Part model, mm, in its own coordinate system. A direction names the side the tool comes from. Round coordinates to 2 decimals unless told otherwise and drop trailing zeros. Loops run counter-clockwise (first coordinate to the right, second up) from the corner with the lowest first, then second, coordinate; pieces in that order, holes last.
1) 3-axis set-ups, long thin cutter, end or side, ignore diameter. For faces 4 (the flat face through (302.45, -195.1, -14.95)), 5 (the flat face through (304.884, -195.453, -28.203)): which of +Z, -Z, +X, -X, +Y, -Y reach the whole face in a straight line?
2) Band-saw the part on C-C, the plane y = -201.5. Write the cut outline in (x, z), then the cut area to 3 significant figures.
3) Band-saw the part on A-A, the plane z = -4. Write the cut outline in (x, y).
4) Probe line 1 (X direction, y = -198.75, z = -15.5); line 2 (X direction, y = -191.75, z = -21.5); line 3 (Z direction, x = 314, y = -187.75). List the from-to ranges inside material, lowest first.
5) Band-saw the part on B-B, the plane z = -17.5. Write the cut outline in (x, y).
6) Drop flat-ended pins along their axis: P1, Ø10, axis at y = -191, z = -7, coming from the +X side; P2, Ø8, axis at x = 329, y = -199.5, coming from the -Z side; P3, Ø6, axis at x = 318, y = -192, coming from the +Z side. Give the stop position or say it passes through.
7) Band-saw the part on D-D, the plane x = 308. Write the cut outline in (y, z), then the cut area to 3 significant figures.
8) Mould opens along X. For faces 1 (the flat face through (321.5, -182.575, -20.2)), 2 (the flat face through (302.59, -195.1, -25.1)), 3 (the flat face through (302.786, -195.453, -10.139)) say: +X half, -X half, draft (parallel to the pull), parting line (faces both ways), or undercut.
Autodesk Inventor part; units mm, degrees
ref_plane "YZ Plane" through (0, 0, 0) normal (1, 0, 0) x (0, 1, 0)
ref_plane "XZ Plane" through (0, 0, 0) normal (0, 1, 0) x (-1, 0, 0)
ref_plane "XY Plane" through (0, 0, 0) normal (0, 0, 1) x (1, 0, 0)
ref_plane "Work Plane1" through (330.6234, -207.9752, -19.9742) normal (0, 1, 0) x (-1, 0, -0.0009)
sketch "Sketch1" plane through (330.6234, -207.9752, -19.9742) normal (0, 1, 0) x (-1, 0, -0.0009)
  circle A0 centre (33.1445, -22.86) radius 4
  circle A1 centre (33.1445, -22.86) radius 4
  circle A2 centre (33.1445, -22.86) radius 4
  line L0 (20.4234, -0.007) -> (20.405, 19.993)
  line L1 (660.8047, 20.5832) -> (0.405, 19.9746)
  line L2 (0.4234, -0.0254) -> (0.405, 19.9746)
  line L3 (0.4234, -0.0254) -> (660.8231, 0.5832)
  line L4 (660.8047, 20.5832) -> (660.8231, 0.5832)
  line L5 (0.405, 19.9746) -> (-7.215, 19.9746)
  line L6 (0.405, 19.9746) -> (0.4234, -0.0254)
  line L7 (0.4234, -0.0254) -> (20.4234, -0.007)
  line L8 (20.4234, -0.007) -> (20.405, 19.993)
  line L9 (35.0462, 0.0065) -> (20.405, 19.993)
  line L10 (-7.215, 19.9746) -> (-7.215, 0.0065)
  line L11 (-7.215, 0.0065) -> (-7.215, -5.0735)
  line L12 (-7.215, -5.0735) -> (20.405, -5.0735)
  line L13 (20.405, -5.0735) -> (31.2395, -11.4268)
  arc A3 (35.0462, -19.341) -> (31.2395, -19.3428) centre (33.1445, -22.86) ccw
  line L14 (31.2395, -19.3428) -> (31.2395, -11.4268)
  line L15 (35.0462, -19.341) -> (35.0462, 0.0065)
  line L16 (20.405, 19.993) -> (20.4234, -0.007)
  line L17 (0.4234, -0.0254) -> (20.4234, -0.007)
  point P0 (330.6048, 20.2789)
  dimension "d0" = 7.62
  dimension "d3" = 5.08
extrude "Extrusion1" add sketch "Sketch1" along normal blind 25.4 contours A0 L14 L13 L12 L11 L10 L5 L2 L3 L15 | L3 L0 L9
sketch "Sketch2" plane through (337.8431, -207.9752, -25.0411) normal (1, 0, 0.0009) x (0.0009, 0, -1)
  line L0 (14.2693, 0) -> (14.2693, 25.4)
  line L1 (-5.0481, 0) -> (-5.0481, 25.4)
  line L2 (-25.0481, 25.4) -> (0, 25.4)
  line L3 (-25.0481, 0) -> (-25.0481, 25.4)
  line L4 (-5.0481, 25.4) -> (-25.0481, 25.4)
  line L5 (-15.0481, 25.4) -> (-15.0481, 12.7)
  circle A0 centre (-15.0481, 12.7) radius 2.5
  point P0 (-25.3524, 207.9752)
  dimension "d6" = 5
extrude "Extrusion2" cut sketch "Sketch2" against normal blind 25.4
sketch "Sketch3" plane through (330.6234, -182.5752, -19.9742) normal (0, 1, 0) x (1, 0, 0.0009)
  line L0 (-20.4234, 0.007) -> (-0.4234, 0.0254)
  line L1 (-0.4234, 0.0254) -> (-0.405, -19.9746)
  line L2 (-0.405, -19.9746) -> (7.215, -19.9746)
  line L3 (7.215, -19.9746) -> (7.215, 5.0735)
  line L4 (7.215, 5.0735) -> (-20.405, 5.0735)
  line L5 (-20.405, 5.0735) -> (-31.2395, 11.4268)
  line L6 (-31.2395, 11.4268) -> (-31.2395, 19.3428)
  arc A0 (-35.0462, 19.341) -> (-31.2395, 19.3428) centre (-33.1445, 22.86) ccw
  line L7 (-35.0462, 19.341) -> (-35.0462, -0.0065)
  line L8 (-35.0462, -0.0065) -> (-20.405, -19.993)
  line L9 (-20.405, -19.993) -> (-20.4234, 0.007)
  line L10 (-32.7964, 8.2501) -> (-32.7964, 0.8179)
  line L11 (-32.7964, 0.8179) -> (-23.4059, -11.0873)
  line L12 (-23.4059, -11.0873) -> (-23.4059, 2.0332)
  line L13 (-23.4059, 2.0332) -> (-32.7964, 8.2501)
  point P0 (-330.6048, -20.2789)
extrude "Extrusion3" cut sketch "Sketch3" against normal blind 50.8 contours L13 L12 L11 L10
sketch "Sketch4" plane through (337.82, -207.9752, 0.007) normal (-0.0009, 0, 1) x (1, 0, 0.0009)
  point P0 (-337.8199, 207.9752)
sketch "Sketch5" plane through (330.6234, -182.5752, -19.9742) normal (0, 1, 0) x (1, 0, 0.0009)
  line L0 (-0.405, -19.9746) -> (7.215, -19.9746)
  line L1 (-0.4234, 0.0254) -> (-0.405, -19.9746)
  line L2 (-0.405, -19.9746) -> (-1.675, -19.9746)
  line L3 (-0.405, -19.9746) -> (0.865, -19.9746) construction
  line L4 (-1.675, -19.9746) -> (0.1211, -21.7706)
  line L5 (0.1211, -21.7706) -> (7.215, -21.7706)
  line L6 (7.215, -21.7706) -> (7.215, -19.9746)
  line L7 (-0.405, -19.9746) -> (-0.405, -19.9746)
  line L8 (-0.405, -19.9746) -> (7.215, -19.9746)
  point P0 (-330.6048, -20.2789)
  dimension "d11" = 1.27
  dimension "d12" = 180
  dimension "d13" = 2.54
  dimension "d14" = 45
extrude "Extrusion4" add sketch "Sketch5" against normal up to surface (25.4 mm away)
properties part number "Braces"
Reported:
1. face 4: +Y, -Y
1. face 5: -Z, +X, +Y, -Y
2. outline: (295.58, -20) - (295.59, -39.35) arc R4 cw to (299.4, -39.35) - (299.39, -31.43) - (310.22, -25.07) - (337.84, -25.04) - (337.82, 1.8) - (330.72, 1.8) - (328.93, 0) - (330.2, 0) - (330.2, -20) - (310.2, -20) - (310.2, 0) - close; hole (297.83, -28.25) - (307.22, -22.03) - (307.21, -8.91) - (297.83, -20.82) - close
2. area: 518 mm2
3. outline: (307.28, -207.98) - (310.2, -207.98) - (310.2, -182.58) - (307.28, -182.58) - close; (330.2, -207.98) - (337.82, -207.98) - (337.82, -182.58) - (330.2, -182.58) - close
4. line 1: x = 298.87 to 302.02, 307.21 to 310.2, 330.2 to 337.83
4. line 2: x = 295.58 to 297.83, 307.22 to 337.84
4. line 3: z = -25.06 to -20
5. outline: (297.4, -207.98) - (300.44, -207.98) - (300.44, -182.58) - (297.4, -182.58) - close; (307.22, -207.98) - (310.2, -207.98) - (310.2, -182.58) - (307.22, -182.58) - close; (330.2, -207.98) - (337.84, -207.98) - (337.84, -182.58) - (330.2, -182.58) - close
6. P1: stops at x = 337.83
6. P2: stops at z = -25.05
6. P3: stops at z = -20
7. outline: (-207.98, -26.37) - (-182.58, -26.37) - (-182.58, -3.01) - (-207.98, -3.01) - close
7. area: 593 mm2
8. face 1: draft
8. face 2: undercut
8. face 3: -X half
